from build123d import *

# Parameters (mm, degrees)
CHAMFER1_SIZE      = 0.625
CUT_EXTRUDE1_DEPTH = 4
CHAMFER2_SIZE      = 0.8
FILLET1_R          = 0.4


with BuildPart() as part:
    # Sketch1 → Revolve1 (revolve)
    with BuildSketch(Plane(origin=(0, 0, 0), x_dir=(1, 0, 0), z_dir=(0, 1, 0))):
        Polygon((0, 0), (0, 4), (5, 4), (5, 2), (20, 2), (20, 0), align=None)
    revolve(axis=Axis((20, 0, 0), (-1, 0, 0)))

    # Chamfer1
    chamfer1_edges = [part.edges().sort_by_distance(p)[0] for p in [
        (20, 0, 2),
    ]]
    chamfer(chamfer1_edges, length=CHAMFER1_SIZE)

    # Sketch3 → Cut-Revolve1 (revolve, cut)
    with BuildSketch(Plane(origin=(0, 0, 0), x_dir=(1, 0, 0), z_dir=(0, 1, 0)), mode=Mode.PRIVATE) as cut_revolve1_sk:
        Polygon((0, 0), (5.732050808, 0), (4, 3), (0, 3), align=None)
    revolve(cut_revolve1_sk.sketch.rotate(Axis((0, 0, 0), (1, 0, 0)), 180), axis=Axis((0, 0, 0), (1, 0, 0)), mode=Mode.SUBTRACT)

    # Sketch2 → Cut-Extrude1 (cut)
    with BuildSketch(Plane.ZY):
        Polygon((0, 3.464101615), (-3, 1.732050808), (-3, -1.732050808), (0, -3.464101615), (3, -1.732050808), (3, 1.732050808), align=None)
    extrude(amount=-CUT_EXTRUDE1_DEPTH, mode=Mode.SUBTRACT)

    # Chamfer2
    # the kernel refuses this chamfer: 0.8 mm, written as the material it takes off along each edge
    with BuildSketch(Plane(origin=(0, 0, 0), x_dir=(0, 0, -1), z_dir=(0, 1, 0))) as chamfer2_piece_1:
        Polygon((4, -CHAMFER2_SIZE), (4 - CHAMFER2_SIZE, 0), (4, 0), align=None)
    revolve(axis=Axis((0, 0, 0), (-1, 0, 0)), mode=Mode.SUBTRACT)

    # Fillet1
    fillet1_edges = [part.edges().sort_by_distance(p)[0] for p in [
        (5, 0, 2),
    ]]
    fillet(fillet1_edges, radius=FILLET1_R)


solid = part.part
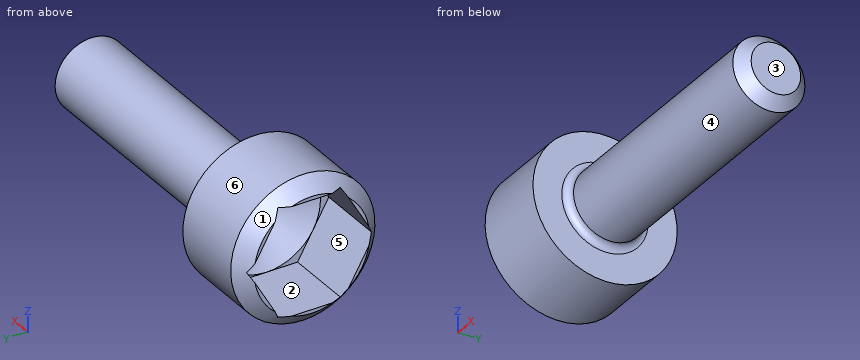
For this review, take the finished solid that the model builds, in its own axes (mm). Face numbers are marked on the shaded views. A direction names the side the tool comes from. Give positions to 0.01 mm unless a question says otherwise; leave off trailing zeros. Loops run counter-clockwise (first coordinate to the right, second up) from the corner with the lowest first, then second, coordinate; pieces in that order, holes last.
Item 1: Tool access review of the marked faces 4, 5 and 6: name each direction out of +Z, -Z, +X, -X, +Y, -Y from which nothing blocks a thin tool from reaching the whole face with its end or side.
Item 2: Take a section at A-A, the plane x = 3. State the section outline as (y, z) points.
Item 3: For line 1 along Z through (x, y) = (2.5, -1.25); line 2 along Y through (x, z) = (1.5, 1); line 3 along Z through (x, y) = (1.75, -1.75), list the stretches that pass through material, from the lowest coordinate up.
Item 4: Insertion check: pin 1 (0.8 mm diameter, centred on y = -1, z = -2, fed in from -X); pin 2 (1.2 mm diameter, centred on y = 1.5, z = -2, fed in from -X); pin 3 (1.7 mm diameter, centred on x = 3, y = -0.5, fed in from +Z); pin 4 (4 mm diameter, centred on x = 13, z = -2.5, fed in from -Y). Each pin has a flat end and moves straight along its axis. Give the tip position at first contact, or say it passes through.
Item 5: Take a section at B-B, the plane x = 19. State the section outline as (y, z) points.
Item 6: Draft analysis for pull direction Z (two halves, no side actions). For the marked faces 1, 2 and 3, state which applies: +Z half, -Z half, draft (parallel to the pull), parting line (faces both ways), or undercut.
Calculated:
1. face 4: +X
1. face 5: -X
1. face 6: +X, -X
2. outline: circle Ø8 at (0, 0); hole (-3.46, 0) - (-1.73, -3) - (1.73, -3) - (3.46, 0) - (1.73, 3) - (-1.73, 3) - close
3. line 1: z = -3.8 to -3, 3 to 3.8
3. line 2: y = -3.87 to -2.89, 2.89 to 3.87
3. line 3: z = -3.6 to -2.97, 2.97 to 3.6
4. pin 1: stops at x = 4.21
4. pin 2: stops at x = 4
4. pin 3: stops at z = 4
4. pin 4: stops at y = -1.94
5. outline: circle Ø4 at (0, 0)
6. face 1: parting line
6. face 2: undercut
6. face 3: draft
